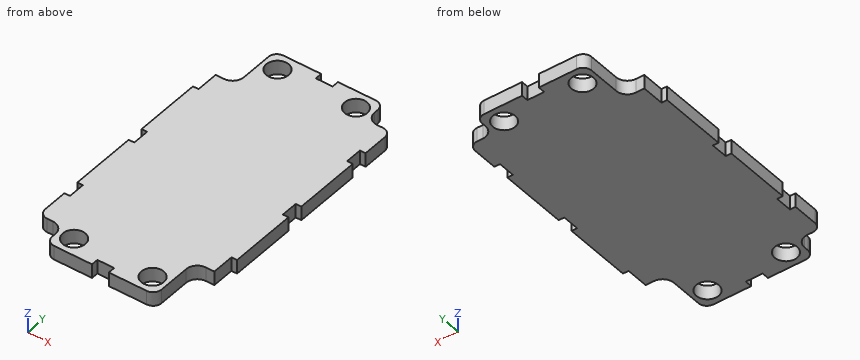
from build123d import *

# Parameters (mm, degrees)
BOX002_W               = 9
BOX002_H               = 9
BOX002_DEPTH           = 10
BOX003_W               = 9
BOX003_H               = 19
BOX003_DEPTH           = 10
BOX004_W               = 9
BOX004_H               = 9
BOX004_DEPTH           = 10
BOX005_W               = 2
BOX005_H               = 6
BOX005_DEPTH           = 10
BOX006_W               = 2
BOX006_H               = 8
BOX006_DEPTH           = 10
BOX007_W               = 2
BOX007_H               = 6
BOX007_DEPTH           = 10
BOX008_W               = 2
BOX008_H               = 6
BOX008_DEPTH           = 10
BOX009_W               = 2
BOX009_H               = 6
BOX009_DEPTH           = 10
BOX010_W               = 2
BOX010_H               = 8
BOX010_DEPTH           = 10
CYLINDER_R             = 4
CYLINDER_DEPTH         = 10
CYLINDER002_R          = 4
CYLINDER002_DEPTH      = 10
CYLINDER001_R          = 4
CYLINDER001_DEPTH      = 10
CYLINDER003_R          = 4
CYLINDER003_DEPTH      = 10
BOX011_W               = 3
BOX011_H               = 6
BOX011_DEPTH           = 10
BOX011_PLACEMENT_ANGLE = 90
BOX012_W               = 3
BOX012_H               = 6
BOX012_DEPTH           = 10
BOX012_PLACEMENT_ANGLE = 90
BOX001_W               = 9
BOX001_H               = 19
BOX001_DEPTH           = 10
BOX_W                  = 57
BOX_H                  = 107
BOX_DEPTH              = 5
FILLET_R               = 3
FILLET001_R            = 4


with BuildPart() as cube002:
    # Box002 → Box002 (new body)
    with BuildSketch(Plane.XY):
        with Locations((4.5, 4.5)):
            Rectangle(BOX002_W, BOX002_H)
    extrude(amount=BOX002_DEPTH)


with BuildPart() as cube003:
    # Box003 → Box003 (new body)
    with BuildSketch(Plane(origin=(0, 89, 0), x_dir=(1, 0, 0), z_dir=(0, 0, 1))):
        with Locations((4.5, 9.5)):
            Rectangle(BOX003_W, BOX003_H)
    extrude(amount=BOX003_DEPTH)


with BuildPart() as cube004:
    # Box004 → Box004 (new body)
    with BuildSketch(Plane(origin=(48, 99, 0), x_dir=(1, 0, 0), z_dir=(0, 0, 1))):
        with Locations((4.5, 4.5)):
            Rectangle(BOX004_W, BOX004_H)
    extrude(amount=BOX004_DEPTH)


with BuildPart() as cube005:
    # Box005 → Box005 (new body)
    with BuildSketch(Plane(origin=(0, 51, 0), x_dir=(1, 0, 0), z_dir=(0, 0, 1))):
        with Locations((1, 3)):
            Rectangle(BOX005_W, BOX005_H)
    extrude(amount=BOX005_DEPTH)


with BuildPart() as cube006:
    # Box006 → Box006 (new body)
    with BuildSketch(Plane(origin=(0, 81, 0), x_dir=(1, 0, 0), z_dir=(0, 0, 1))):
        with Locations((1, 4)):
            Rectangle(BOX006_W, BOX006_H)
    extrude(amount=BOX006_DEPTH)


with BuildPart() as cube007:
    # Box007 → Box007 (new body)
    with BuildSketch(Plane(origin=(0, 21, 0), x_dir=(1, 0, 0), z_dir=(0, 0, 1))):
        with Locations((1, 3)):
            Rectangle(BOX007_W, BOX007_H)
    extrude(amount=BOX007_DEPTH)


with BuildPart() as cube008:
    # Box008 → Box008 (new body)
    with BuildSketch(Plane(origin=(55, 51, 0), x_dir=(1, 0, 0), z_dir=(0, 0, 1))):
        with Locations((1, 3)):
            Rectangle(BOX008_W, BOX008_H)
    extrude(amount=BOX008_DEPTH)


with BuildPart() as cube009:
    # Box009 → Box009 (new body)
    with BuildSketch(Plane(origin=(55, 81, 0), x_dir=(1, 0, 0), z_dir=(0, 0, 1))):
        with Locations((1, 3)):
            Rectangle(BOX009_W, BOX009_H)
    extrude(amount=BOX009_DEPTH)


with BuildPart() as cube010:
    # Box010 → Box010 (new body)
    with BuildSketch(Plane(origin=(55, 19, 0), x_dir=(1, 0, 0), z_dir=(0, 0, 1))):
        with Locations((1, 4)):
            Rectangle(BOX010_W, BOX010_H)
    extrude(amount=BOX010_DEPTH)


with BuildPart() as cylinder:
    # Cylinder → Cylinder (new body)
    with BuildSketch(Plane(origin=(14.5, 6.5, 0), x_dir=(1, 0, 0), z_dir=(0, 0, 1))):
        Circle(CYLINDER_R)
    extrude(amount=CYLINDER_DEPTH)


with BuildPart() as cylinder002:
    # Cylinder002 → Cylinder002 (new body)
    with BuildSketch(Plane(origin=(42.5, 101.5, 0), x_dir=(1, 0, 0), z_dir=(0, 0, 1))):
        Circle(CYLINDER002_R)
    extrude(amount=CYLINDER002_DEPTH)


with BuildPart() as cylinder001:
    # Cylinder001 → Cylinder001 (new body)
    with BuildSketch(Plane(origin=(42.5, 6.5, 0), x_dir=(1, 0, 0), z_dir=(0, 0, 1))):
        Circle(CYLINDER001_R)
    extrude(amount=CYLINDER001_DEPTH)


with BuildPart() as cylinder003:
    # Cylinder003 → Cylinder003 (new body)
    with BuildSketch(Plane(origin=(14.5, 101.5, 0), x_dir=(1, 0, 0), z_dir=(0, 0, 1))):
        Circle(CYLINDER003_R)
    extrude(amount=CYLINDER003_DEPTH)


with BuildPart() as cube011:
    # Box011 → Box011 (new body)
    with BuildSketch(Plane.XY):
        with Locations((1.5, 3)):
            Rectangle(BOX011_W, BOX011_H)
    extrude(amount=BOX011_DEPTH)


with BuildPart() as cube011_1:
    # Box011 placement: moved
    add(cube011.part.moved(Location((31.5, 0, 0))).rotate(Axis((31.5, 0, 0), (0, 0, 1)), BOX011_PLACEMENT_ANGLE))


with BuildPart() as cube012:
    # Box012 → Box012 (new body)
    with BuildSketch(Plane.XY):
        with Locations((1.5, 3)):
            Rectangle(BOX012_W, BOX012_H)
    extrude(amount=BOX012_DEPTH)


with BuildPart() as cube012_1:
    # Box012 placement: moved
    add(cube012.part.moved(Location((31.5, 105, 0))).rotate(Axis((31.5, 105, 0), (0, 0, 1)), BOX012_PLACEMENT_ANGLE))


with BuildPart() as fusion:
    # Box001 → Box001 (new body)
    with BuildSketch(Plane(origin=(48, 0, 0), x_dir=(1, 0, 0), z_dir=(0, 0, 1))):
        with Locations((4.5, 9.5)):
            Rectangle(BOX001_W, BOX001_H)
    extrude(amount=BOX001_DEPTH)

    # Fusion: union Cube002, Cube003, Cube004, Cube005, Cube006, Cube007, Cube008, Cube009, Cube010, Cylinder, Cylinder002, Cylinder001, Cylinder003, Cube011, Cube012
    add(cube002.part)
    add(cube003.part)
    add(cube004.part)
    add(cube005.part)
    add(cube006.part)
    add(cube007.part)
    add(cube008.part)
    add(cube009.part)
    add(cube010.part)
    add(cylinder.part)
    add(cylinder002.part)
    add(cylinder001.part)
    add(cylinder003.part)
    add(cube011_1.part)
    add(cube012_1.part)


with BuildPart() as fillet001:
    # Box → Box (new body)
    with BuildSketch(Plane(origin=(0, 0.5, 0), x_dir=(1, 0, 0), z_dir=(0, 0, 1))):
        with Locations((28.5, 53.5)):
            Rectangle(BOX_W, BOX_H)
    extrude(amount=BOX_DEPTH)

    # Cut: cut Fusion
    add(fusion.part, mode=Mode.SUBTRACT)

    # Fillet
    fillet_edges = [fillet001.edges().sort_by_distance(p)[0] for p in [
        (9, 107.5, 2.5),
        (48, 107.5, 2.5),
        (57, 99, 2.5),
        (48, 0.5, 2.5),
        (9, 0.5, 2.5),
        (0, 9, 2.5),
    ]]
    fillet(fillet_edges, radius=FILLET_R)

    # Fillet001
    fillet001_edges = [fillet001.edges().sort_by_distance(p)[0] for p in [
        (9, 89, 2.5),
        (48, 99, 2.5),
        (9, 9, 2.5),
        (48, 19, 2.5),
    ]]
    fillet(fillet001_edges, radius=FILLET001_R)


solid = fillet001.part
Geometry: final body of the model. Coordinates: model frame, mm. Coordinates: 2 decimals unless noted, no trailing zeros. Loops run counter-clockwise (first coordinate to the right, second up) from the corner with the lowest first, then second, coordinate; pieces in that order, holes last. Notation, with made-up numbers: (-23, 12) - (-12, 12) arc R13 ccw to (-12, 33) - close; hole circle Ø4 at (46.5, 5.25). An arc over 180 degrees is marked (long way). Put each result on its own line as item: value. Start each with the question number.
Q1. Cut plane C-C, the plane z = 1.5. Give the number of separate pieces and of enclosed holes in the cut face, and give its area (3 significant figures).
Q2. Cut plane B-B, the plane y = 101.5. Return loops of the section in (x, z).
Q3. Cut plane D-D, the plane y = 53. Return loops of the section in (x, z), and give its area (3 significant figures).
Q4. Cut plane A-A, the plane x = 42.5. Return loops of the section in (y, z), and give its area (3 significant figures).
Q5. Pin query (flat end, axial travel): pin 1 Ø7 at (x, y) = (14.5, 101.5) entering from -Z; pin 2 Ø2 at (y, z) = (1.5, 3) entering from +X; pin 3 Ø2 at (x, z) = (55.5, 3) entering from +Y; pin 4 Ø1.6 at (x, z) = (56, 2) entering from +Y. Return the tip coordinate at first contact, or that it passes through.
Q6. Line query: line 1 (Y direction, x = 42.5, z = 2.5); line 2 (X direction, y = 6.5, z = 3.95); line 3 (X direction, y = 99.5, z = 1.8). Output: solid intervals per line, ascending.
Filled sheet:
1. separate pieces: 1
1. enclosed holes: 4
1. area: 5,300 mm²
2. outline: (9, 0) - (10.5, 0) - (10.5, 5) - (9, 5) - close; (18.5, 0) - (38.5, 0) - (38.5, 5) - (18.5, 5) - close; (46.5, 0) - (48.29, 0) - (48.29, 5) - (46.5, 5) - close
3. outline: (2, 0) - (55, 0) - (55, 5) - (2, 5) - close
3. area: 265 mm²
4. outline: (0.5, 0) - (2.5, 0) - (2.5, 5) - (0.5, 5) - close; (10.5, 0) - (97.5, 0) - (97.5, 5) - (10.5, 5) - close; (105.5, 0) - (107.5, 0) - (107.5, 5) - (105.5, 5) - close
4. area: 455 mm²
5. pin 1: through
5. pin 2: x = 47.83
5. pin 3: y = 98.96
5. pin 4: y = 98.75
6. line 1: 0.5 to 2.5, 10.5 to 97.5, 105.5 to 107.5
6. line 2: 8.71 to 10.5, 18.5 to 38.5, 46.5 to 48
6. line 3: 9 to 11.04, 17.96 to 39.04, 45.96 to 50.06
